The figure shows three views and two pictorial views of one solid part (mm, origin at its lowest corner). Answer the questions. Coordinates: 2 decimals unless noted, no trailing zeros. Write each loop counter-clockwise with the first axis right and the second up, starting at its lowest first coordinate (ties: lowest second). Pieces come first, ordered by that corner, then holes. Notation, with made-up numbers: M 73.5,-11 L 131.5,-11 A33 ccw 131.5,22 Z; hole C 83.25,82.5 d1. An arc over 180 degrees is marked long. Use CSV: the item, a comma, the result in double quotes.
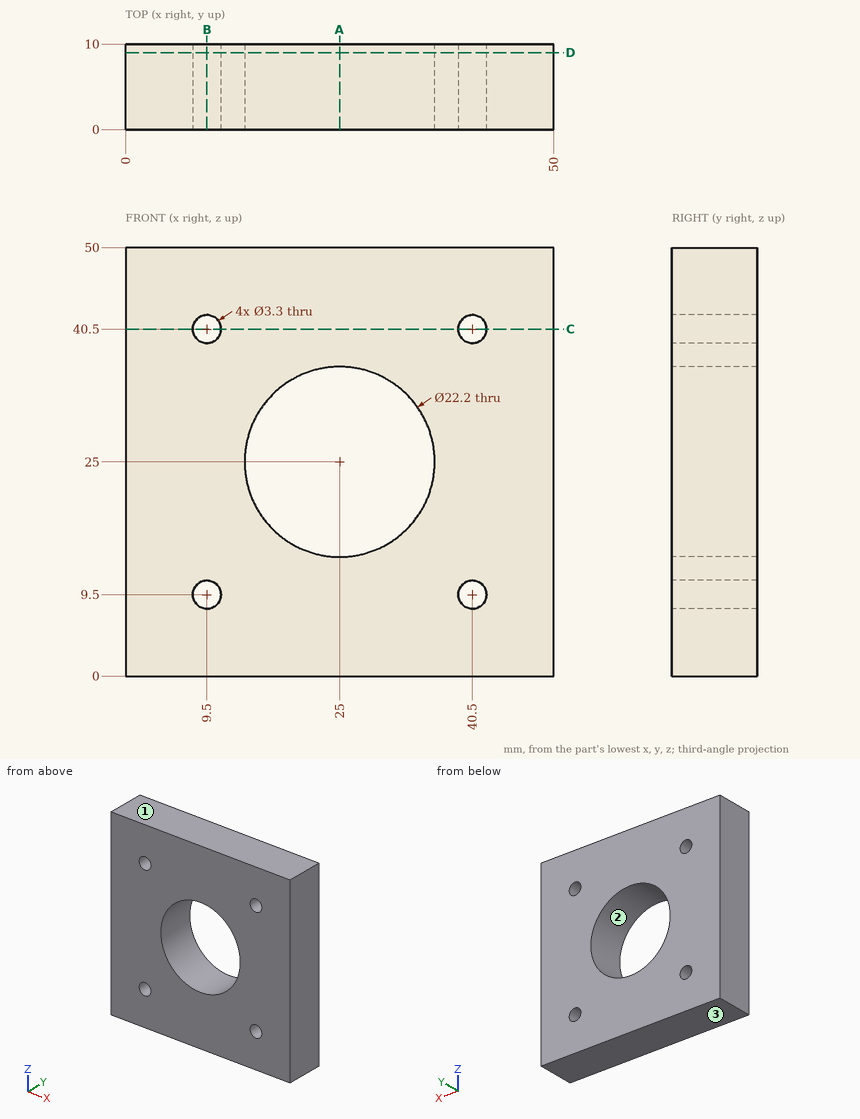
Item 1: The part is cut by section B-B (x = 9.5). Write down the section's boundary in (y, z).
Answer:
outline,"M 0,0 L 10,0 L 10,7.85 L 0,7.85 Z; M 0,11.15 L 10,11.15 L 10,38.85 L 0,38.85 Z; M 0,42.15 L 10,42.15 L 10,50 L 0,50 Z"
Item 2: Consider probe 1 along Z at (x, y) = (40.5, 6); probe 2 along X at (y, z) = (1.25, 8). Determine where each line is inside the solid, lowest interval first.
Answer:
probe 1,"z = 0 to 7.85, 11.15 to 38.85, 42.15 to 50"
probe 2,"x = 0 to 8.81, 10.19 to 39.81, 41.19 to 50"
Item 3: The part is cut by section D-D (y = 9). Write down the section's boundary in (x, z), then the cut area to 3 significant figures.
Answer:
outline,"M 0,0 L 50,0 L 50,50 L 0,50 Z; hole C 9.5,9.5 d3.3; hole C 9.5,40.5 d3.3; hole C 25,25 d22.2; hole C 40.5,9.5 d3.3; hole C 40.5,40.5 d3.3"
area,"2,080 mm2"
Item 4: For a pull along Z with two mould halves and no side action, classify the marked faces 1, 2 and 3 as released by +Z, released by -Z, zero draft, split by the parting line, or undercut.
Answer:
face 1,"released by +Z"
face 2,"undercut"
face 3,"released by -Z"
Item 5: Given pin 1 (1 mm diameter, centred on x = 36, y = 3.5, fed in from -Z), flat-ended and moving along its own axis, determine where the tip first touches the part or whether it passes through.
Answer:
pin 1,"stops at z = 0"
Item 6: The part is cut by section A-A (x = 25). Write down the section's boundary in (y, z).
Answer:
outline,"M 0,0 L 10,0 L 10,13.9 L 0,13.9 Z; M 0,36.1 L 10,36.1 L 10,50 L 0,50 Z"
Item 7: The part is cut by section C-C (z = 40.5). Write down the section's boundary in (x, y), then the cut area to 3 significant figures.
Answer:
outline,"M 0,0 L 7.85,0 L 7.85,10 L 0,10 Z; M 11.15,0 L 38.85,0 L 38.85,10 L 11.15,10 Z; M 42.15,0 L 50,0 L 50,10 L 42.15,10 Z"
area,"434 mm2"
